Autodesk Inventor part; units mm, degrees
ref_plane "YZ Plane" through (0, 0, 0) normal (1, 0, 0) x (0, 1, 0)
ref_plane "XZ Plane" through (0, 0, 0) normal (0, 1, 0) x (-1, 0, 0)
ref_plane "XY Plane" through (0, 0, 0) normal (0, 0, 1) x (1, 0, 0)
sketch "スケッチ1" plane through (0, 0, 0) normal (0, 1, 0) x (-1, 0, 0)
  line L0 (0, 0) -> (204, 0)
  line L1 (204, 0) -> (204, -72)
  line L2 (204, -72) -> (0, -72)
  line L3 (0, -72) -> (0, 0)
  dimension "d0" = 204
  dimension "d1" = 72
extrude "押し出し1" add sketch "スケッチ1" along normal blind 7
sketch "スケッチ2" plane through (0, 7, 0) normal (0, 1, 0) x (1, 0, 0)
  line L0 (-204, 22) -> (-112, 22)
  line L1 (-112, 22) -> (-112, 72)
  line L2 (-112, 72) -> (-204, 72)
  line L3 (-204, 72) -> (-204, 22)
  line L4 (-204, 72) -> (-204, 0)
  line L5 (0, 72) -> (-204, 72)
  line L6 (-204, 0) -> (0, 0)
  dimension "d5" = 92
  dimension "d76" = 50
extrude "押し出し2" cut sketch "スケッチ2" against normal through all
sketch "スケッチ3" plane through (0, 7, 0) normal (0, 1, 0) x (1, 0, 0)
  line L0 (-204, 22) -> (-204, 0)
  line L1 (-204, 22) -> (-112, 22)
  line L2 (-112, 22) -> (-112, 14)
  line L3 (-112, 14) -> (-204, 14)
  line L4 (-204, 14) -> (-204, 22)
  line L5 (-112, 72) -> (-112, 22)
  line L6 (-112, 72) -> (-104, 72)
  line L7 (-104, 72) -> (-104, 14)
  line L8 (-104, 14) -> (-112, 14)
  line L9 (-112, 14) -> (-112, 72)
  line L10 (0, 72) -> (-112, 72)
  line L11 (0, 0) -> (0, 72)
  line L12 (-112, 72) -> (0, 72)
  line L13 (0, 72) -> (0, 64)
  line L14 (0, 64) -> (-112, 64)
  line L15 (-112, 64) -> (-112, 72)
  point P0 (-204, 14)
  point P1 (-104, 64)
  dimension "d8" = 8
  dimension "d9" = 8
  dimension "d19" = 8
extrude "押し出し3" cut sketch "スケッチ3" against normal blind 4
sketch "スケッチ4" plane through (0, 3, 0) normal (0, 1, 0) x (1, 0, 0)
  circle A0 centre (-192, 18) radius 1.5
  circle A1 centre (-108, 18) radius 1.5
  circle A2 centre (-108, 59) radius 1.5
  line L0 (-112, 72) -> (0, 72)
  line L1 (-204, 14) -> (-204, 22)
  line L2 (-112, 22) -> (-112, 72)
  circle A3 centre (-88, 68) radius 1.5
  circle A4 centre (-12, 68) radius 1.5
  line L3 (0, 72) -> (0, 64)
  point P0 (0, 0)
  point P1 (-204, 18)
  point P2 (-204, 18)
  dimension "d12" = 3
  dimension "d13" = 3
  dimension "d14" = 3
  dimension "d16" = 12
  dimension "d20" = 4
  dimension "d21" = 3
  dimension "d22" = 3
  dimension "d23" = 4
  dimension "d24" = 24
  dimension "d25" = 12
  dimension "d32" = 41
  dimension "d34" = 76
extrude "押し出し4" cut sketch "スケッチ4" against normal through all
sketch "スケッチ5" plane through (0, 0, 0) normal (0, -1, 0) x (1, 0, 0)
  line L0 (-204, 0) -> (0, 0)
  line L1 (-204, -22) -> (-112, -22)
  line L2 (-204, 0) -> (-196, 0)
  line L3 (-196, 0) -> (-196, -22)
  line L4 (-196, -22) -> (-204, -22)
  line L5 (-204, -22) -> (-204, 0)
  dimension "d26" = 8
extrude "押し出し5" cut sketch "スケッチ5" against normal blind 2
sketch "スケッチ6" plane through (0, 0, 0) normal (0, -1, 0) x (1, 0, 0)
  line L0 (-196, 0) -> (-196, -22)
  line L1 (0, 0) -> (-196, 0)
  line L2 (-196, 0) -> (-196, -5)
  line L3 (-196, -5) -> (0, -5)
  line L4 (0, -5) -> (0, 0)
  line L5 (-196, 0) -> (0, 0)
  line L6 (-112, -72) -> (0, -72)
  line L7 (0, 0) -> (-5, 0)
  line L8 (-5, 0) -> (-5, -72)
  line L9 (-5, -72) -> (0, -72)
  line L10 (0, -72) -> (0, 0)
  point P0 (0, -72)
  point P1 (-5, -5)
  dimension "d29" = 5
  dimension "d33" = 5
extrude "押し出し6" add sketch "スケッチ6" along normal blind 55
fillet "フィレット1" radius 2 4 edges at (-102, 7, 0) (0, 7, -32) (0, -24, 0) (-204, 7, -7)
sketch "スケッチ7" plane through (-5, 0, -5) normal (0, 0, -1) x (-1, 0, 0)
  line L0 (191, 2) -> (191, -55)
  line L1 (0, 0) -> (191, 0)
  line L2 (191, -55) -> (181, -55)
  line L3 (181, -55) -> (181, 0)
  line L4 (181, 0) -> (191, 0)
  line L5 (191, 0) -> (191, -55)
  point P0 (-5, 0)
  dimension "d36" = 10
extrude "押し出し7" add sketch "スケッチ7" along normal blind 3
sketch "スケッチ8" plane through (-196, 2, -22) normal (-1, 0, 0) x (0, 0, 1)
  circle A0 centre (18, -41) radius 1.5
  circle A1 centre (18, -8) radius 1.5
  line L0 (22, -57) -> (14, -57)
  line L1 (0, 0) -> (22, 0)
  point P0 (22, -2)
  point P1 (18, -57)
  point P2 (18, -57)
  dimension "d39" = 3
  dimension "d40" = 3
  dimension "d41" = 16
  dimension "d62" = 8
extrude "押し出し8" cut sketch "スケッチ8" against normal blind 8
sketch "スケッチ9" plane through (0, -55, 0) normal (0, -1, 0) x (1, 0, 0)
  line L0 (-5, -5) -> (-5, -72)
  circle A0 centre (-5, -5) radius 3
  circle A1 centre (-5, -64) radius 3
  line L1 (-186, -5) -> (-5, -5)
  circle A2 centre (-101, -5) radius 3
  circle A3 centre (-191, -5) radius 3
  line L2 (-5, -72) -> (0, -72)
  point P0 (0, 0)
  dimension "d45" = 6
  dimension "d46" = 6
  dimension "d47" = 6
  dimension "d48" = 96
  dimension "d49" = 6
  dimension "d50" = 90
  dimension "d78" = 8
extrude "押し出し9" add sketch "スケッチ9" against normal blind 15 contours L1 A0 L0 | L0 A0 L1 | A1 L0 | L0 A1 | A2 L1 | L1 A2
sketch "スケッチ10" plane through (0, -55, 0) normal (0, -1, 0) x (1, 0, 0)
  line L0 (-5, -5) -> (-186, -5)
  circle A0 centre (-5, -5) radius 1.5
  line L1 (-98, -5) -> (-104, -5)
  circle A1 centre (-101, -5) radius 1.5
  arc A2 (-5, -61) -> (-5, -67) centre (-5, -64) ccw
  circle A3 centre (-5, -64) radius 1.5
  circle A4 centre (-189, -5) radius 1.5
  line L2 (-186, -8) -> (-196, -8)
  line L3 (-186, -5) -> (-186, -8)
  point P0 (0, 0)
  dimension "d54" = 3
  dimension "d55" = 3
  dimension "d56" = 3
  dimension "d57" = 3
  dimension "d58" = 3
  dimension "d59" = 3
extrude "押し出し10" cut sketch "スケッチ10" against normal blind 12
sketch "スケッチ11" plane through (0, 7, 0) normal (0, 1, 0) x (1, 0, 0)
  circle A0 centre (-198.5, 10) radius 2.8
  line L0 (-204, 14) -> (-204, 0)
  line L1 (-204, 0) -> (-2, 0)
  line L2 (-104, 14) -> (-202, 14)
  line L3 (-202, 2) -> (-202, 14)
  point P0 (0, 0)
  dimension "d63" = 5.6
  dimension "d65" = 5.5
  dimension "d77" = 4
  dimension "d79" = 10
extrude "押し出し11" cut sketch "スケッチ11" against normal blind 2.5
sketch "スケッチ12" plane through (-198.5, 4.5, -10) normal (0, 1, 0) x (1, 0, 0)
  line L0 (2.5, -10) -> (2.5, 12)
  circle A0 centre (0, 0) radius 1.5
  circle A1 centre (0, 0) radius 2.8
  point P0 (198.5, -10)
  dimension "d71" = 3
extrude "押し出し12" cut sketch "スケッチ12" against normal through all contours A0
fillet "フィレット2" radius 2 2 edges at (-203.4142, 6.4142, -0.5858) (-204, 3.5, 0)
properties part number "オンゲキボタン_top1_3D プリント"
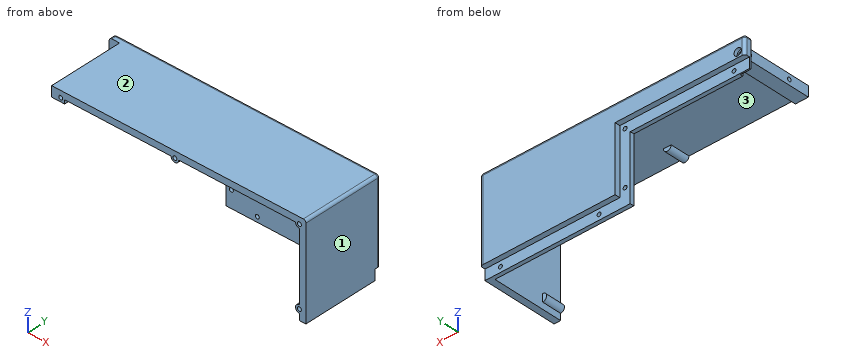
Input: part model. Units: mm. Frame: model coordinates. Face numbers are marked on the shaded views. Coordinates: 2 decimals unless noted, no trailing zeros. Write each loop counter-clockwise with the first axis right and the second up, starting at its lowest first coordinate (ties: lowest second). Pieces come first, ordered by that corner, then holes. Notation, with made-up numbers: M -37.5,62.5 L -25.5,62.5 A34 ccw -25.5,96.5 Z; hole C -17,48 d4. An arc over 180 degrees is marked long. Answer as a JSON object with one key per item and string values. Group by question number.
(1) Ray query, line 1 along X through (y, z) = (1.05, -18); line 2 along Z through (x, y) = (-12, 1.3); line 3 along Z through (x, y) = (-108, 1.75). Return the intervals inside material, ascending. Write a range as [from, to].
(2) Contact query for flat-ended pins moving along their axis: P1, Ø2.5, axis at y = -39, z = -3.5, coming from the -X side; P2, Ø1.5, axis at y = -41, z = -6.5, coming from the +X side; P3, Ø3, axis at x = -89.5, y = -40.5, coming from the -Z side; P4, Ø2.5, axis at x = -201.5, z = -8, coming from the -Y side. Output: stop coordinate, or through.
(3) Section B-B on x = -143.5. Output: boundary loops of the cut face in (y, z).
(4) Section A-A on y = -30. Output: boundary loops of the cut face in (x, z).
(5) Mould query, pull axis X, two halves, no side actions, for the marked faces 1, 2 and 3. Classes: pulls with the +X half, pulls with the -X half, needs draft (parallel to the pull), parting line crosses it, or undercut.
Result set:
{
 "1": {"line 1": "x = [-196, -193.5], [-190.5, -109.5], [-106.5, 0]", "line 2": "z = [-72, -69.5], [-66.5, 0]", "line 3": "z = [-72, -60.5], [-57.5, -19.5], [-16.5, 0]"},
 "2": {"P1": "stops at x = -196", "P2": "stops at x = 0", "P3": "stops at z = -5", "P4": "stops at y = 2"},
 "3": {"outline": "M -55,-5 L 0,-5 L 0,-22 L 3,-22 L 3,-14 L 7,-14 L 7,-2 A2 ccw 5,0 L -55,0 Z"},
 "4": {"outline": "M -196,-8 L -186,-8 L -186,-5 L -5,-5 L -5,-72 L 0,-72 L 0,-2 A2 ccw -2,0 L -196,0 Z"},
 "5": {"face 1": "pulls with the +X half", "face 2": "needs draft", "face 3": "undercut"}
}
